Source: three-view drawing plus pictorial views. Frame: mm from the lowest corner of the part. Round coordinates to 2 decimals unless told otherwise and drop trailing zeros. Loops run counter-clockwise (first coordinate to the right, second up) from the corner with the lowest first, then second, coordinate; pieces in that order, holes last. Notation, with made-up numbers: (-1, 10) -> (55, 10) arc R17 cw to (55, 20) -> close; hole circle Ø10 at (2.25, 25). An arc over 180 degrees is marked (long way). Answer in a Markdown table with one row per item. Add a question column.
Q1. Section A-A, the plane x = 14.75. Output: boundary loops of the cut face in (y, z).
Q2. Section C-C, the plane y = 9. Output: boundary loops of the cut face in (x, z), and give its area (3 significant figures).
Q3. Ray query, L1, parallel to Y at x = 16, z = 1.15; L2, parallel to Y at x = 9, z = 1.25; L3, parallel to X at y = 1.5, z = 0.85. Return the intervals inside material, ascending. Write a range as from..to.
Q4. Mould query, pull axis X, two halves, no side actions, for the marked faces 1, 2 and 3. Classes: pulls with the +X half, pulls with the -X half, needs draft (parallel to the pull), parting line crosses it, or undercut.
Q5. Section D-D, the plane x = 16.75. Output: boundary loops of the cut face in (y, z).
Q6. Section B-B, the plane z = 0.4. Output: boundary loops of the cut face in (x, y), and give its area (3 significant figures).
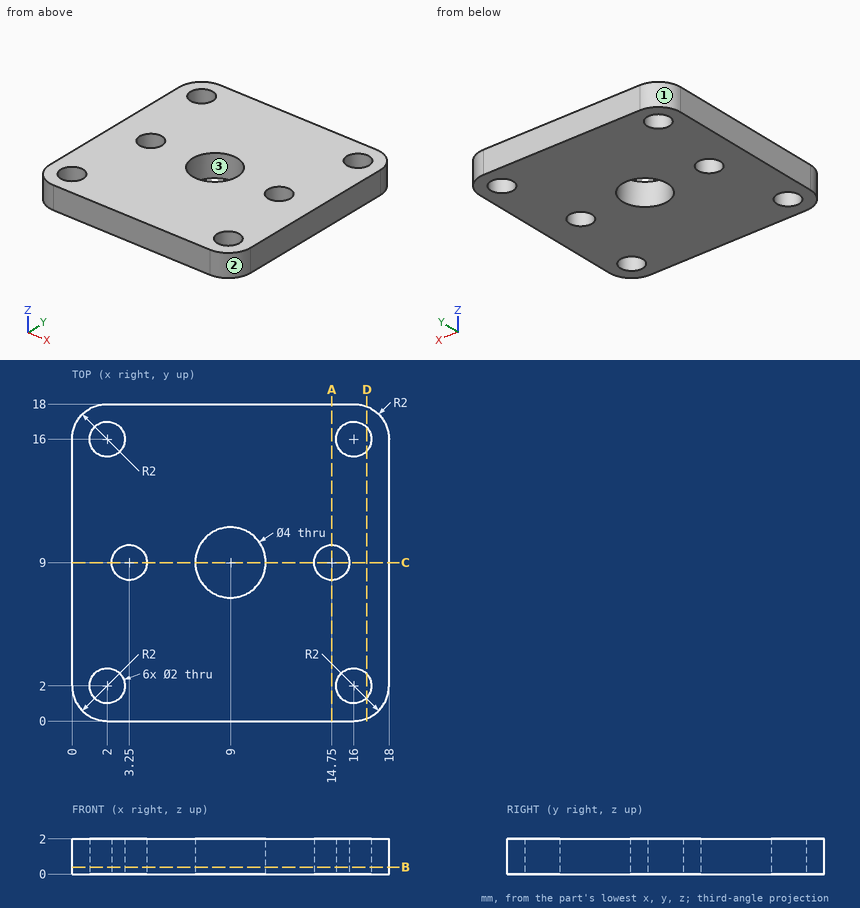
Answer block:
| question | item | result |
|---|---|---|
| 1 | outline | (0, 0) -> (8, 0) -> (8, 2) -> (0, 2) -> close; (10, 0) -> (18, 0) -> (18, 2) -> (10, 2) -> close |
| 2 | outline | (0, 0) -> (2.25, 0) -> (2.25, 2) -> (0, 2) -> close; (4.25, 0) -> (7, 0) -> (7, 2) -> (4.25, 2) -> close; (11, 0) -> (13.75, 0) -> (13.75, 2) -> (11, 2) -> close; (15.75, 0) -> (18, 0) -> (18, 2) -> (15.75, 2) -> close |
| 2 | area | 20.0 mm^2 |
| 3 | L1 | 0..1, 3..15, 17..18 |
| 3 | L2 | 0..7, 11..18 |
| 3 | L3 | 0.06..1.13, 2.87..15.13, 16.87..17.94 |
| 4 | face 1 | pulls with the -X half |
| 4 | face 2 | pulls with the +X half |
| 4 | face 3 | undercut |
| 5 | outline | (0.15, 0) -> (1.34, 0) -> (1.34, 2) -> (0.15, 2) -> close; (2.66, 0) -> (15.34, 0) -> (15.34, 2) -> (2.66, 2) -> close; (16.66, 0) -> (17.85, 0) -> (17.85, 2) -> (16.66, 2) -> close |
| 6 | outline | (0, 2) arc R2 ccw to (2, 0) -> (16, 0) arc R2 ccw to (18, 2) -> (18, 16) arc R2 ccw to (16, 18) -> (2, 18) arc R2 ccw to (0, 16) -> close; hole circle Ø2 at (2, 2); hole circle Ø2 at (2, 16); hole circle Ø2 at (3.25, 9); hole circle Ø4 at (9, 9); hole circle Ø2 at (14.75, 9); hole circle Ø2 at (16, 2); hole circle Ø2 at (16, 16) |
| 6 | area | 289 mm^2 |
